Geometry: final body of the model. Coordinates: model frame, mm. Face numbers are marked on the shaded views. Round coordinates to 2 decimals unless told otherwise and drop trailing zeros. Loops run counter-clockwise (first coordinate to the right, second up) from the corner with the lowest first, then second, coordinate; pieces in that order, holes last. Notation, with made-up numbers: M 72.25,68 L 98.25,68 A18 ccw 98.25,85 Z; hole C 42.5,26 d8. An arc over 180 degrees is marked long. Answer as a JSON object with one key per item and string values.
```python
from build123d import *

# Parameters (mm, degrees)
BASE_FLANGE1_DEPTH = 88.2
CHAMFER1_SIZE      = 5
FILLET1_R          = 2.5
SKETCH4_R          = 4
CUT_EXTRUDE1_DEPTH = 92.368703613
SKETCH5_R          = 1.25
CUT_EXTRUDE2_DEPTH = 92.368703613
SKETCH6_R          = 1.25
CUT_EXTRUDE3_DEPTH = 98.361388651


# Sheet-metal steps are written as plain solids
with BuildPart() as part:
    # Sketch1 → Base-Flange1 (new body)
    with BuildSketch(Plane.XY):
        with BuildLine():
            Line((10, -17), (3, -17))
            ThreePointArc((3, -17), (0.878679656, -16.121320344), (0, -14))
            Line((0, -14), (0, 0))
            Line((0, 0), (0, 14))
            ThreePointArc((0, 14), (0.878679656, 16.121320344), (3, 17))
            Line((3, 17), (10, 17))
            Line((10, 17), (10, 20))
            Line((10, 20), (3, 20))
            ThreePointArc((3, 20), (-1.242640687, 18.242640687), (-3, 14))
            Line((-3, 14), (-3, 0))
            Line((-3, 0), (-3, -14))
            ThreePointArc((-3, -14), (-1.242640687, -18.242640687), (3, -20))
            Line((3, -20), (10, -20))
            Line((10, -20), (10, -17))
        make_face()
    extrude(amount=BASE_FLANGE1_DEPTH)

    # Chamfer1
    chamfer1_edges = [part.edges().sort_by_distance(p)[0] for p in [
        (10, 18.5, 0),
        (10, -18.5, 0),
        (10, 18.5, 88.2),
        (10, -18.5, 88.2),
    ]]
    chamfer(chamfer1_edges, length=CHAMFER1_SIZE)

    # Fillet1
    fillet1_edges = [part.edges().sort_by_distance(p)[0] for p in [
        (5, -18.5, 0),
        (10, -18.5, 83.2),
        (10, -18.5, 5),
        (5, 18.5, 0),
        (10, 18.5, 83.2),
        (10, 18.5, 5),
        (5, -18.5, 88.2),
        (5, 18.5, 88.2),
    ]]
    fillet(fillet1_edges, radius=FILLET1_R)

    # Sketch4 → Cut-Extrude1 (cut, through all)
    with BuildSketch(Plane.ZY.offset(3)):
        with Locations(Location((44.1, 0, 0), (0, 0, 270))):
            Circle(SKETCH4_R)
    extrude(amount=-CUT_EXTRUDE1_DEPTH, mode=Mode.SUBTRACT)

    # Sketch5 → Cut-Extrude2 (cut, through all)
    with BuildSketch(Plane.ZY.offset(3)):
        with Locations(Location((44.1, 11, 0), (0, 0, 270))):
            Circle(SKETCH5_R)
        with Locations(Location((51.878174593, 7.778174593, 0), (0, 0, 270))):
            Circle(SKETCH5_R)
        with Locations(Location((55.1, 0, 0), (0, 0, 270))):
            Circle(SKETCH5_R)
        with Locations(Location((51.878174593, -7.778174593, 0), (0, 0, 270))):
            Circle(SKETCH5_R)
        with Locations(Location((44.1, -11, 0), (0, 0, 270))):
            Circle(SKETCH5_R)
        with Locations(Location((36.321825407, -7.778174593, 0), (0, 0, 270))):
            Circle(SKETCH5_R)
        with Locations(Location((33.1, 0, 0), (0, 0, 270))):
            Circle(SKETCH5_R)
        with Locations(Location((36.321825407, 7.778174593, 0), (0, 0, 270))):
            Circle(SKETCH5_R)
    extrude(amount=-CUT_EXTRUDE2_DEPTH, mode=Mode.SUBTRACT)

    # Sketch6 → Cut-Extrude3 (cut, through all)
    with BuildSketch(Plane(origin=(0, 20, 0), x_dir=(1, 0, 0), z_dir=(0, 1, 0))):
        with Locations(Location((7.2, -79.1, 0), (0, 0, 270))):
            Circle(SKETCH6_R)
        with Locations(Location((7.2, -58.1, 0), (0, 0, 270))):
            Circle(SKETCH6_R)
        with Locations(Location((7.2, -30.1, 0), (0, 0, 90))):
            Circle(SKETCH6_R)
        with Locations(Location((7.2, -9.1, 0), (0, 0, 90))):
            Circle(SKETCH6_R)
    extrude(amount=-CUT_EXTRUDE3_DEPTH, mode=Mode.SUBTRACT)


solid = part.part
```
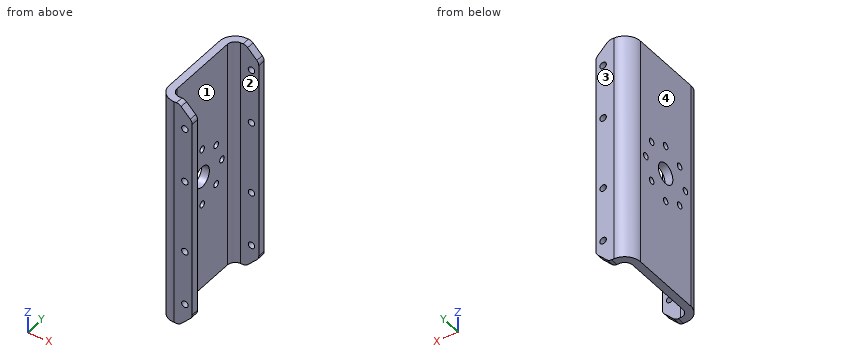
1) Cut plane A-A on z = 79.1. Return the cut outline in (x, y), and give its area (3 significant figures).
Geometry results:
{"outline": "M -3,-14 A6 ccw 3,-20 L 5.95,-20 L 5.95,-17 L 3,-17 A3 cw 0,-14 L 0,14 A3 cw 3,17 L 5.95,17 L 5.95,20 L 3,20 A6 ccw -3,14 Z; M 8.45,-20 L 10,-20 L 10,-17 L 8.45,-17 Z; M 8.45,17 L 10,17 L 10,20 L 8.45,20 Z", "area": "153 mm2"}
2) Cut plane D-D on x = 1. Return the cut outline in (y, z), and give its area (3 significant figures).
Geometry results:
{"outline": "M -19.66,0 L -16.24,0 L -16.24,88.2 L -19.66,88.2 Z; M 16.24,0 L 19.66,0 L 19.66,88.2 L 16.24,88.2 Z", "area": "603 mm2"}
3) First-contact query: pin 1 (22.5 mm diameter, centred on y = 3.5, z = 39, fed in from +X); pin 2 (3 mm diameter, centred on y = 2.5, z = 24, fed in from +X). Flat tips, straight axial feed; report the tip coordinate or a pass-through.
Geometry results:
{"pin 1": "x = 0.1", "pin 2": "x = 0"}
4) Cut plane B-B on y = 0. Return the cut outline in (x, z).
Geometry results:
{"outline": "M -3,0 L 0,0 L 0,31.85 L -3,31.85 Z; M -3,34.35 L 0,34.35 L 0,40.1 L -3,40.1 Z; M -3,48.1 L 0,48.1 L 0,53.85 L -3,53.85 Z; M -3,56.35 L 0,56.35 L 0,88.2 L -3,88.2 Z"}
5) Cut plane C-C on z = 55.1. Return the cut outline in (x, y).
Geometry results:
{"outline": "M -3,-14 A6 ccw 3,-20 L 10,-20 L 10,-17 L 3,-17 A3 cw 0,-14 L 0,-1.25 L -3,-1.25 Z; M -3,1.25 L 0,1.25 L 0,14 A3 cw 3,17 L 10,17 L 10,20 L 3,20 A6 ccw -3,14 Z"}
6) Line query: probe 1 along Y at (x, z) = (8, 13.5); probe 2 along Z at (x, y) = (-0.5, -8); probe 3 along Y at (x, z) = (-0.5, 53). Output: solid intervals per line, ascending.
Geometry results:
{"probe 1": "-20 to -17, 17 to 20", "probe 2": "0 to 35.09, 37.55 to 50.65, 53.11 to 88.2", "probe 3": "-18.87 to -8.33, -7.23 to 7.23, 8.33 to 18.87"}
7) Pull-direction query (Y, two-part tool) for the marked faces 1, 2, 3 and 4; classes: +Y half, -Y half, draft (parallel to the pull), parting line (faces both ways), or undercut.
Geometry results:
{"face 1": "undercut", "face 2": "undercut", "face 3": "+Y half", "face 4": "draft"}
